```python
from build123d import *

# Parameters (mm, degrees)
F0_R     = 7.5
F0_R_2   = 4
F1_DEPTH = 5


with BuildPart() as f1:
    # F0 (on Front) → F1 (new body)
    with BuildSketch(Plane.XZ):
        with BuildLine():
            Line((-39, -9.949874), (0.6, -5.969925))
            ThreePointArc((0.6, -5.969925), (6, 0), (0.6, 5.969925))
            Line((0.6, 5.969925), (-39, 9.949874))
            ThreePointArc((-39, 9.949874), (-50, 0), (-39, -9.949874))
        make_face()
        with Locations((-40, 0)):
            Circle(F0_R, mode=Mode.SUBTRACT)
        Circle(F0_R_2, mode=Mode.SUBTRACT)
    extrude(amount=F1_DEPTH)


solid = f1.part
```
Work out the finished part from the listing and answer in its coordinate system (mm). Give positions to 0.01 mm unless a question says otherwise; leave off trailing zeros. Loops run counter-clockwise (first coordinate to the right, second up) from the corner with the lowest first, then second, coordinate; pieces in that order, holes last. Notation, with made-up numbers: (-29, 40.25) -> (5, 40.25) arc R23 cw to (5, 60.25) -> close; hole circle Ø11 at (88.25, 28). An arc over 180 degrees is marked (long way). Use CSV: the item, a comma, the result in double quotes.
1. The mould has two halves that part along X. Classify faces 1 (the cylindrical face through (-0.867, -2.465, -3.905)), 2 (the flat face through (-18.92, -2.46, 7.93)), 3 (the flat face through (-22, 0, 0)): +X half, -X half, draft (parallel to the pull), parting line (faces both ways), or undercut.
Found:
face 1,"undercut"
face 2,"+X half"
face 3,"draft"
2. The part is cut by section D-D (z = -3.25). Write down the section's boundary in (x, y), then the cut area to 3 significant figures.
Found:
outline,"(-49.46, -5) -> (-46.76, -5) -> (-46.76, 0) -> (-49.46, 0) -> close; (-33.24, -5) -> (-2.33, -5) -> (-2.33, 0) -> (-33.24, 0) -> close; (2.33, -5) -> (5.04, -5) -> (5.04, 0) -> (2.33, 0) -> close"
area,"182 mm^2"
3. The part is cut by section B-B (x = -40). Write down the section's boundary in (y, z).
Found:
outline,"(-5, -10) -> (0, -10) -> (0, -7.5) -> (-5, -7.5) -> close; (-5, 7.5) -> (0, 7.5) -> (0, 10) -> (-5, 10) -> close"
4. The part is cut by section A-A (z = 0). Write down the section's boundary in (x, y).
Found:
outline,"(-50, -5) -> (-47.5, -5) -> (-47.5, 0) -> (-50, 0) -> close; (-32.5, -5) -> (-4, -5) -> (-4, 0) -> (-32.5, 0) -> close; (4, -5) -> (6, -5) -> (6, 0) -> (4, 0) -> close"
5. Flat-ended cylindrical pins translate along their axes: pin 1 Ø1 at (x, y) = (-38, -2) entering from -Z; pin 2 Ø1.5 at (x, y) = (-12, -2.5) entering from +Z; pin 3 Ø3 at (x, y) = (-8.5, -1.5) entering from -Z. Find the tip coordinate at first contact, or state that the pin passes through.
Found:
pin 1,"z = -9.9"
pin 2,"z = 7.31"
pin 3,"z = -7.04"
6. Straight lines are drawn through the part: line 1 (Z direction, x = -40, y = -1.2); line 2 (X direction, y = -4.8, z = 1.75); line 3 (X direction, y = -0.35, z = 0.25). For each, find the intervals that lie inside material, in ascending order.
Found:
line 1,"-10 to -7.5, 7.5 to 10"
line 2,"-49.85 to -47.29, -32.71 to -3.6, 3.6 to 5.74"
line 3,"-50 to -47.5, -32.5 to -3.99, 3.99 to 5.99"
7. The part is cut by section C-C (y = -4.15). Write down the section's boundary in (x, z).
Found:
outline,"(-39, -9.95) -> (0.6, -5.97) arc R6 ccw to (0.6, 5.97) -> (-39, 9.95) arc R10 ccw (long way) to start; hole circle Ø15 at (-40, 0); hole circle Ø8 at (0, 0)"
